```python
from build123d import *

# Parameters (mm, degrees)
REVOLVE_1_ANGLE     = 180
CUT_EXTRUDE_1_REACH = 179.268
SKETCH_26_W         = 11
SKETCH_26_H         = 9.4
SKETCH_30_W         = 159
SKETCH_30_H         = 71.5
EXTRUDE_3_DEPTH     = 10
EXTRUDE_4_REACH     = 203.503
SKETCH_31_R         = 5


# Read off the part's stored shape, not the designer's step: the revolve step
with BuildPart() as part:
    # Sweep 1: sweep along a path in Sketch 1
    with BuildLine(Plane(origin=(0, 0, 0), x_dir=(0, 0, -1), z_dir=(1, 0, 0))) as sweep_1_path:
        Line((0, 0), (80, -6.999093082))
    # Sketch 8 → Sweep 1 (sweep)
    with BuildSketch(Plane.XY):
        with BuildLine():
            Line((5, 0), (7.5, 0))
            Line((7.5, 0), (7.5, -8))
            Line((7.5, -8), (-7.5, -8))
            Line((-7.5, -8), (-7.5, 0))
            Line((-7.5, 0), (-5, 0))
            ThreePointArc((-5, 0), (0, -5), (5, 0))
        make_face()
    sweep(path=sweep_1_path.line)

    # Sweep 2: sweep along a path in Sketch 3
    with BuildLine(Plane(origin=(0, -6.999093082, 0), x_dir=(1, 0, 0), z_dir=(0, 1, 0))) as sweep_2_path:
        ThreePointArc((0, 80), (-2.928932188, 87.071067812), (-10, 90))
    # Sketch 15 → Sweep 2 (sweep)
    with BuildSketch(Plane(origin=(0, 0, -80), x_dir=(-1, 0, 0), z_dir=(0, 0, -1))):
        with BuildLine():
            Line((7.5, -14.999093082), (7.5, -6.999093082))
            Line((7.5, -6.999093082), (5, -6.999093082))
            ThreePointArc((5, -6.999093082), (0, -11.999093082), (-5, -6.999093082))
            Line((-5, -6.999093082), (-7.5, -6.999093082))
            Line((-7.5, -6.999093082), (-7.5, -14.999093082))
            Line((-7.5, -14.999093082), (7.5, -14.999093082))
        make_face()
    sweep(path=sweep_2_path.line)

    # Sweep 6: sweep along a path in Sketch 4
    with BuildLine(Plane.XY.offset(-90)) as sweep_6_path:
        ThreePointArc((-114, -55), (-85.48557321, -45.758350859), (-65, -23.876351309))
        ThreePointArc((-65, -23.876351309), (-59.344635199, -19.169851161), (-52, -19.606461369))
        ThreePointArc((-52, -19.606461369), (-43.328947167, -20.827564341), (-35.453602253, -16.999093082))
        ThreePointArc((-35.453602253, -16.999093082), (-23.673751019, -9.588764492), (-10, -6.999093082))
    # Sketch 19 → Sweep 6 (sweep)
    with BuildSketch(Plane.ZY.offset(10)):
        with BuildLine():
            Line((-97.5, -14.999093082), (-82.5, -14.999093082))
            Line((-82.5, -14.999093082), (-82.5, -6.999093082))
            Line((-82.5, -6.999093082), (-85, -6.999093082))
            ThreePointArc((-85, -6.999093082), (-90, -11.999093082), (-95, -6.999093082))
            Line((-95, -6.999093082), (-97.5, -6.999093082))
            Line((-97.5, -6.999093082), (-97.5, -14.999093082))
        make_face()
    sweep(path=sweep_6_path.line)

    # Sweep 7: sweep along a path in Sketch 5
    with BuildLine(Plane(origin=(0, -55, 0), x_dir=(1, 0, 0), z_dir=(0, 1, 0))) as sweep_7_path:
        ThreePointArc((-114, 90), (-121.071067812, 87.071067812), (-124, 80))
    # Sketch 20 → Sweep 7 (sweep)
    with BuildSketch(Plane(origin=(-116.921360423, -7.136292944, 0), x_dir=(0, 0, 1), z_dir=(-0.9981425535898466, -0.06092161121589024, 0))):
        with BuildLine():
            Line((-97.5, -47.952776769), (-97.5, -55.952776769))
            Line((-97.5, -55.952776769), (-82.5, -55.952776769))
            Line((-82.5, -55.952776769), (-82.5, -47.952776769))
            Line((-82.5, -47.952776769), (-85, -47.952776769))
            ThreePointArc((-85, -47.952776769), (-90, -52.952776769), (-95, -47.952776769))
            Line((-95, -47.952776769), (-97.5, -47.952776769))
        make_face()
    sweep(path=sweep_7_path.line)

    # Sweep 8: sweep along a path in Sketch 6
    with BuildLine(Plane(origin=(-124, 0, 0), x_dir=(0, 0, -1), z_dir=(1, 0, 0))) as sweep_8_path:
        Line((80, -55), (1.557937214, -59.902628924))
        ThreePointArc((1.557937214, -59.902628924), (-0.000760155, -59.975651302), (-1.560977094, -60))
        Line((-1.560977094, -60), (-17, -60))
    # Sketch 21 → Sweep 8 (sweep)
    with BuildSketch(Plane(origin=(0, 4.660546858, -76.358619691), x_dir=(1, 0, 0), z_dir=(0, -0.06092161121589024, 0.9981425535898466))):
        with BuildLine():
            Line((-129, -59.771569345), (-131.5, -59.771569345))
            Line((-131.5, -59.771569345), (-131.5, -67.771569345))
            Line((-131.5, -67.771569345), (-116.5, -67.771569345))
            Line((-116.5, -67.771569345), (-116.5, -59.771569345))
            Line((-116.5, -59.771569345), (-119, -59.771569345))
            ThreePointArc((-119, -59.771569345), (-124, -64.771569345), (-129, -59.771569345))
        make_face()
    sweep(path=sweep_8_path.line)

    # Sweep 9: sweep along a path in Sketch 22
    with BuildLine(Plane(origin=(0, 0, 0), x_dir=(1, 0, 0), z_dir=(0, 1, 0))) as sweep_9_path:
        ThreePointArc((0, 0), (-2.928932188, -7.071067812), (-10, -10))
    # Sketch 23 → Sweep 9 (sweep)
    with BuildSketch(Plane.XY):
        with BuildLine():
            Line((-7.5, 0), (-7.5, -8))
            Line((-7.5, -8), (7.5, -8))
            Line((7.5, -8), (7.5, 0))
            Line((7.5, 0), (5, 0))
            ThreePointArc((5, 0), (0, -5), (-5, 0))
            Line((-5, 0), (-7.5, 0))
        make_face()
    sweep(path=sweep_9_path.line)

    # Revolve 1 outline → Revolve 1 (revolve)
    with BuildSketch(Plane(origin=(-124, 0.024682835, 16.912396843), x_dir=(-1, 0, 0), z_dir=(1.4532479245137334e-14, -0.0014594506721384598, -0.9999989350013008))):
        with BuildLine():
            Line((7.5, -68.024746762), (7.5, -60.024746762))
            Line((7.5, -60.024746762), (5, -60.024746762))
            ThreePointArc((5, -60.024746762), (3.535533906, -63.560280668), (0, -65.024746762))
            Line((0, -65.024746762), (0, -68.024746762))
            Line((0, -68.024746762), (7.5, -68.024746762))
        make_face()
    revolve(axis=Axis((-124, 0.024682835, 16.912396843), (0, 0.9999989350013008, -0.0014594506721384598)), revolution_arc=REVOLVE_1_ANGLE)

    # Sketch 26 → Cut-Extrude 1 (cut, up to next)
    with BuildSketch(Plane(origin=(0, 0, 0), x_dir=(1, 0, 0), z_dir=(0, 1, 0)), mode=Mode.PRIVATE) as cut_extrude_1_sk1:
        with Locations((-122, -10.5)):
            Rectangle(SKETCH_26_W, SKETCH_26_H)
    cut_extrude_1_tool1 = extrude(cut_extrude_1_sk1.sketch, amount=-CUT_EXTRUDE_1_REACH, mode=Mode.PRIVATE) & part.part
    add(cut_extrude_1_tool1.solids().sort_by_distance((-122, 0, 10.5))[0], mode=Mode.SUBTRACT)

    # Sketch 31 → Extrude 4 (add, up to next)
    with BuildSketch(Plane(origin=(0, -95, 0), x_dir=(1, 0, 0), z_dir=(0, 1, 0)), mode=Mode.PRIVATE) as extrude_4_sk1:
        with Locations(Location((-121.071067812, 87.071067812, 0), (0, 0, 90))):
            Circle(SKETCH_31_R)
    extrude_4_tool1 = extrude(extrude_4_sk1.sketch, amount=EXTRUDE_4_REACH, mode=Mode.PRIVATE) - part.part
    # Sketch 31 → Extrude 4 (add, up to next)
    with BuildSketch(Plane(origin=(0, -95, 0), x_dir=(1, 0, 0), z_dir=(0, 1, 0)), mode=Mode.PRIVATE) as extrude_4_sk2:
        with Locations(Location((-2.928932188, 87.071067812, 0), (0, 0, 90))):
            Circle(SKETCH_31_R)
    extrude_4_tool2 = extrude(extrude_4_sk2.sketch, amount=EXTRUDE_4_REACH, mode=Mode.PRIVATE) - part.part


with BuildPart() as body_2:
    # Sketch 30 → Extrude 3 (new body)
    with BuildSketch(Plane(origin=(0, -105, 0), x_dir=(-1, 0, 0), z_dir=(0, -1, 0))):
        with Locations((62, 71.75)):
            Rectangle(SKETCH_30_W, SKETCH_30_H)
    extrude(amount=-EXTRUDE_3_DEPTH)


with BuildPart() as part_1:
    add(part.part)

    add(body_2.part)  # Extrude 4 merges body 2
    add(extrude_4_tool1.solids().sort_by_distance((-121.071068, -95, -87.071068))[0])
    add(extrude_4_tool2.solids().sort_by_distance((-2.928932, -95, -87.071068))[0])


solid = part_1.part
```
Verification items for the finished model (mm, model axes). A direction names the side the tool comes from. Give positions to 0.01 mm unless a question says otherwise; leave off trailing zeros. Loops run counter-clockwise (first coordinate to the right, second up) from the corner with the lowest first, then second, coordinate; pieces in that order, holes last. Notation, with made-up numbers: M -7,-2 L 5,-2 A16 ccw 5,15 Z; hole C 16,60 d1. An arc over 180 degrees is marked long. One line per question, with ' | ' between items.
Item 1: Tool access check on faces 1 (the face through (-1, -14.999, -92)), 2 (the face through (-8, -6.999, -82)), 3 (the face through (-10, -6, 10)), 4 (the face through (-116, -55, -82)), 5 (the face through (-81.603, -52.768, -89.895)). Record the directions out of +Z, -Z, +X, -X, +Y, -Y that give a thin tool (end or side, any length) a straight path to the whole face; none if there is none.
Completed:
face 1: none | face 2: -Z, +X, -X, +Y | face 3: +Z, -X, +Y, -Y | face 4: +Z, -Z, -X, +Y | face 5: +Z, -Z
Item 2: Depth check by flat-ended pin: P1, Ø9, axis at y = -3, z = 11, coming from the -X side; P2, Ø4, axis at x = 0.5, z = -34.5, coming from the -Y side; P3, Ø5.5, axis at x = -2.5, z = -87.5, coming from the +Y side; P4, Ø6, axis at x = -14, z = -40.5, coming from the +Y side. Enter the tip coordinate at first touch or a pass-through.
Completed:
P1: stops at x = -10 | P2: stops at y = -105 | P3: stops at y = -10.7 | P4: stops at y = -95
Item 3: Section check A-A, the plane y = -71.5. Record the cut outline in (x, z).
Completed:
outline: C -121.07,-87.07 d10; C -2.93,-87.07 d10
Item 4: Section check B-B, the plane z = -38. State how many separate pieces and enclosed holes the cut face has, plus the area to 3 significant figures.
Completed:
separate pieces: 3 | enclosed holes: 0 | area: 1,750 mm^2
Item 5: Thickness scan on line 1 (Y direction, x = -11, z = -46); line 2 (Y direction, x = -44, z = -90); line 3 (X direction, y = -43.5, z = -83.5). Record the ranges inside material, lowest first. Write a range as [from, to].
Completed:
line 1: y = [-105, -95] | line 2: y = [-105, -95], [-28.95, -25.94] | line 3: x = [-82.18, -69.88], [-6.43, 0.57]
Item 6: Draft check along Y on faces 6 (the face through (-125, -55, -91)), 7 (the face through (-0.1, -11.55, -40.56)), 8 (the face through (-141.5, -100, -71)). Enter one of: +Y half, -Y half, draft (parallel to the pull), parting line (faces both ways), or undercut.
Completed:
face 6: +Y half | face 7: undercut | face 8: draft
